Read the model definition and answer for the solid it produces. Units are mm, in the model's axes. Face numbers are marked on the shaded views. Coordinates: 2 decimals unless noted, no trailing zeros. Order: outer loops, then holes, each group sorted by start corner. A loop starts at its lowest first (then second) coordinate and runs counter-clockwise, first axis right, second up. Notation, with made-up numbers: M -6,-27 L 2,-27 A16 ccw 2,-10 Z; hole C 49,79.25 d2. An arc over 180 degrees is marked long. Put each result on its own line as item: value.
Autodesk Inventor part; units mm, degrees
ref_plane "YZ Plane" through (0, 0, 0) normal (1, 0, 0) x (0, 1, 0)
ref_plane "XZ Plane" through (0, 0, 0) normal (0, 1, 0) x (-1, 0, 0)
ref_plane "XY Plane" through (0, 0, 0) normal (0, 0, 1) x (1, 0, 0)
sketch "スケッチ1" plane through (0, 0, 0) normal (0, 1, 0) x (-1, 0, 0)
  circle A0 centre (0, 0) radius 35
  line L0 (0, 0) -> (0, -35)
  line L1 (0, 0) -> (0, 35)
  dimension "d0" = 70
revolve "回転1" add sketch "スケッチ1" angle 180 about axis through (0, 0, 0) along (0, 0, 1) picked at (-2.5961, -23.0408) contours L1 L0 A0
sketch "スケッチ5" plane through (0, 0, 0) normal (0, -1, 0) x (1, 0, 0)
  line L0 (-20, -22) -> (20, -22)
  line L1 (20, -22) -> (20, -13)
  line L2 (20, -13) -> (-20, -13)
  line L3 (-20, -13) -> (-20, -22)
  line L4 (-20, -15) -> (-20, -13)
  line L5 (0, 25) -> (-17, 25)
  line L6 (-17, 25) -> (-17, 23)
  line L7 (-17, 23) -> (0, 23)
  line L8 (0, 23) -> (0, 25)
  line L9 (0, 20) -> (-20, 20)
  line L10 (-20, 20) -> (-20, 19)
  line L11 (-20, 19) -> (0, 19)
  line L12 (0, 19) -> (0, 20)
  line L13 (0, 13) -> (-19, 13)
  line L14 (-19, 13) -> (-19, 11)
  line L15 (-19, 11) -> (0, 11)
  line L16 (0, 11) -> (0, 13)
  line L17 (0, 5) -> (-23, 5)
  line L18 (-23, 5) -> (-23, 3)
  line L19 (-23, 3) -> (0, 3)
  line L20 (0, 3) -> (0, 5)
  circle A0 centre (0, 0) radius 35
  circle A1 centre (0, 0) radius 35
  line L21 (0, 35) -> (0, -35)
  line L22 (35, 0) -> (-35, 0)
  line L23 (-32, 2) -> (-23, 2)
  line L24 (-23, 2) -> (-23, -8)
  line L25 (-23, -8) -> (-32, -8)
  line L26 (-32, -8) -> (-32, 2)
  line L27 (-23, -8.0262) -> (-23, 2)
  line L28 (-27, 22.2711) -> (-27, -22.2711)
  line L29 (-15.5, 25) -> (0, 25)
  line L30 (0, 25) -> (0, 35)
  line L31 (0, 35) -> (-15.5, 35)
  line L32 (-15.5, 35) -> (-15.5, 25)
  line L33 (-15.5, 23) -> (0, 23)
  line L34 (0, 23) -> (0, 20)
  line L35 (0, 20) -> (-15.5, 20)
  line L36 (-15.5, 20) -> (-15.5, 23)
  line L37 (-16, 13) -> (0, 13)
  line L38 (0, 13) -> (0, 19)
  line L39 (0, 19) -> (-16, 19)
  line L40 (-16, 19) -> (-16, 13)
  line L41 (-16, 11) -> (0, 11)
  line L42 (0, 11) -> (0, 5)
  line L43 (0, 5) -> (-16, 5)
  line L44 (-16, 5) -> (-16, 11)
  line L45 (-23, -3) -> (-39.6865, -3)
  line L46 (-23, -3) -> (-7.8337, -3)
  line L47 (-8, 3) -> (-23, 3)
  line L48 (-23, 3) -> (-23, -9)
  line L49 (-23, -9) -> (-8, -9)
  line L50 (-8, -9) -> (-8, 3)
  line L51 (-8, 3) -> (-23, -9) construction
  line L52 (-23, 3) -> (-8, -9) construction
  line L53 (-23, 4) -> (-33, 4)
  line L54 (-33, 4) -> (-33, -10)
  line L55 (-33, -10) -> (-23, -10)
  line L56 (-23, -10) -> (-23, 4)
  line L57 (-23, 4) -> (-33, -10) construction
  line L58 (-33, 4) -> (-23, -10) construction
  line L59 (-8, 3) -> (-1, 3)
  line L60 (-1, 3) -> (-1, -9)
  line L61 (-1, -9) -> (-8, -9)
  line L62 (-8, -9) -> (-8, 3)
  line L63 (-8, 3) -> (-1, -9) construction
  line L64 (-1, 3) -> (-8, -9) construction
  line L65 (-23, 2) -> (-27, 2)
  line L66 (-23, -8) -> (-27, -8)
  line L67 (-23, 4) -> (-27, 4)
  line L68 (-23, -10) -> (-27, -10)
  line L69 (23.4307, -26) -> (-23.4307, -26)
  line L70 (-8, 3) -> (-6.8, 3)
  line L71 (-6.8, 3) -> (-6.8, -9)
  line L72 (-6.8, -9) -> (-8, -9)
  line L73 (-8, -9) -> (-8, 3)
  line L74 (-3, 5) -> (0, 5)
  line L75 (0, 20) -> (-4, 20)
  line L76 (-4, 19) -> (0, 19)
  line L77 (0, 19) -> (0, 20)
  line L78 (-6, 5) -> (-1, 5)
  line L79 (-1, 3) -> (-6, 3)
  point P0 (0, -22)
  point P1 (0, -13)
  point P2 (0, 24)
  point P3 (0, 19.5)
  point P4 (0, 12)
  point P5 (0, 4)
  point P6 (-20, -17.5)
  point P7 (-27, -0.5262)
  point P8 (-27, -8)
  point P9 (-15.5, 21.5)
  point P10 (-15.5, 31.3807)
  point P11 (0, 25)
  point P12 (0, 23)
  point P13 (0, 11)
  point P14 (0, 13)
  point P15 (-27, 0)
  point P16 (-32, 0)
  point P17 (-23, 0)
  point P18 (-15.5, -3)
  point P19 (-28, -3)
  point P20 (-4.5, -3)
  point P21 (-8, -9)
  point P22 (-8, 3)
  point P23 (-27, 0.5)
  point P24 (-28, 0.4738)
  point P25 (-28, -11.5262)
  point P26 (-27, -11.5)
  point P27 (-23, 2)
  point P28 (-23, 2)
  point P29 (-8, 0)
  point P30 (-1, 0)
  point P31 (0, 19)
  point P32 (0, 20)
  point P33 (-27, -10)
  point P34 (-27, 4)
  dimension "d12" = 40
  dimension "d13" = 9
  dimension "d23" = 17
  dimension "d24" = 2
  dimension "d27" = 20
  dimension "d28" = 1
  dimension "d30" = 19
  dimension "d31" = 2
  dimension "d33" = 2
  dimension "d88" = 0
  dimension "d89" = 0
  dimension "d90" = 13
  dimension "d92" = 20
  dimension "d93" = 10
  dimension "d97" = 9
  dimension "d98" = 10
  dimension "d113" = 27
  dimension "d122" = 15.5
  dimension "d123" = 35
  dimension "d124" = 3
  dimension "d125" = 15.5
  dimension "d126" = 6
  dimension "d127" = 6
  dimension "d128" = 16
  dimension "d129" = 16
  dimension "d147" = 12
  dimension "d149" = 8
  dimension "d151" = 15
  dimension "d161" = 14
  dimension "d162" = 10
  dimension "d164" = 12
  dimension "d165" = 7
  dimension "d170" = 26
  dimension "d175" = 1.2
  dimension "d207" = 0
extrude "GNSボード" cut sketch "スケッチ5" against normal blind 16 contours L8 L7 L6 L5
extrude "GNSボード止めるよう" cut sketch "スケッチ5" against normal blind 15 contours L21 L5 L32 A0 | L21 L9 L36 L7
extrude "アルミ板１" cut sketch "スケッチ5" against normal blind 17.5 contours L11 L10 L9 L12
extrude "メイン基板" cut sketch "スケッチ5" against normal blind 17.5 contours L15 L14 L13 L16
extrude "メイン止めるよう" cut sketch "スケッチ5" against normal blind 16.5 contours L17 L44 L15 L21 | L13 L40 L11 L21
extrude "アルミ板２" cut sketch "スケッチ5" against normal blind 19 contours L19 L18 L17 L20
extrude "電池ボックス入れ" cut sketch "スケッチ5" against normal blind 15 contours L3 L2 L21 L0 | L21 L2 L1 L0
extrude "side ut" cut sketch "スケッチ5" against normal blind 100 contours A0 L45 L54 L55 L28 | A0 L22 L54 L45 | L55 L54 L45 L26 L25 L28 | A0 L28 L53 L54 L22 | L54 L22 L26 L45 | L25 L26 L45 L28 | L54 L53 L28 L23 L26 L22 | L26 L22 L28 L45 | L22 L26 L23 L28
extrude "motor case" add sketch "スケッチ5" against normal blind 7 contours L55 L54 L45 L26 L25 L28 | L28 L25 L27 L48 L56 L55 | L50 L46 L24 L22 | L22 L24 L48 L19 L50 | L54 L22 L26 L45 | L28 L45 L24 L25 | L25 L26 L45 L28 | L24 L45 L28 L22 | L22 L28 L23 L24 | L50 L49 L48 L27 L24 L46 | L54 L53 L28 L23 L26 L22 | L26 L22 L28 L45 | L53 L18 L48 L23 L28 | L22 L26 L23 L28
extrude "bottom cut" cut sketch "スケッチ5" against normal blind 90 contours L69 A0 L21 | L21 A0 L69
extrude "motor" cut sketch "スケッチ5" against normal blind 6 contours L60 L61 L71 L22 | L22 L71 L19 L60 | L71 L61 L50 L22 | L22 L50 L19 L71 | L50 L46 L24 L22 | L22 L24 L48 L19 L50 | L28 L45 L24 L25 | L25 L26 L45 L28 | L24 L45 L28 L22 | L22 L28 L23 L24 | L50 L49 L48 L27 L24 L46 | L26 L22 L28 L45 | L22 L26 L23 L28
extrude "motor block" add sketch "スケッチ5" against normal blind 10 contours L71 L61 L50 L22 | L22 L50 L19 L71
sketch "スケッチ27" plane through (-33, 0, -10) normal (-1, 0, 0) x (0, 0, 1)
  line L0 (14, 0) -> (0, 0)
  circle A0 centre (7, 0) radius 3
  point P0 (10, 0)
  dimension "d198" = 6
extrude "押し出し36" cut sketch "スケッチ27" against normal blind 27
mirror "ミラー13" about plane through (0, 0, 0) normal (1, 0, 0) of "メイン止めるよう", "メイン基板", "アルミ板１", "GNSボード止めるよう", "GNSボード", "アルミ板２", "motor", "motor case", "押し出し36", "電池ボックス入れ", "side ut"
ref_plane "作業平面5" through (-17, 17.5, 23) normal (0, -1, 0) x (1, 0, 0)
sketch "スケッチ29" plane through (-17, 17.5, 23) normal (0, -1, 0) x (1, 0, 0)
  line L0 (32.5, 2) -> (1.5, 2)
  line L1 (1.5, 0) -> (32.5, 0)
  line L2 (32.5, -3) -> (1.5, -3)
  line L3 (1, -4) -> (33, -4)
  line L4 (33, -10) -> (1, -10)
  line L5 (33, -10) -> (33, -4)
  line L6 (1, -4) -> (33, -4)
  line L7 (1, -10) -> (1, -4)
  line L8 (1, -12) -> (33, -12)
  line L9 (33, -18) -> (1, -18)
  line L10 (33, -18) -> (33, -12)
  line L11 (1, -12) -> (33, -12)
  line L12 (1, -18) -> (1, -12)
  line L13 (18, -20) -> (40, -20)
  line L14 (-6, -20) -> (17, -20)
  line L15 (17, -18) -> (-6, -18)
  line L16 (-16, -23) -> (-15, -23)
  line L17 (-15, -23) -> (-15, -21)
  line L18 (-15, -21) -> (-6, -21)
  line L19 (-6, -21) -> (-6, -18)
  line L20 (-6, -18) -> (1, -18)
  line L21 (1, -18) -> (1, -12)
  line L22 (1, -12) -> (-2, -12)
  line L23 (-2, -12) -> (-2, -10)
  line L24 (-2, -10) -> (1, -10)
  line L25 (1, -10) -> (1, -4)
  line L26 (1, -4) -> (-3, -4)
  line L27 (-3, -4) -> (-3, -3)
  line L28 (-3, -3) -> (1.5, -3)
  line L29 (1.5, -3) -> (1.5, 0)
  line L30 (1.5, 0) -> (0, 0)
  line L31 (0, 0) -> (0, 2)
  line L32 (0, 2) -> (1.5, 2)
  line L33 (1.5, 2) -> (1.5, 8.3807)
  arc A0 (1.5, 8.3807) -> (-10, -0.7289) centre (17, -23) ccw
  line L34 (-10, -0.7289) -> (-10, -19)
  line L35 (-10, -19) -> (-16, -19)
  line L36 (-16, -19) -> (-16, -23)
  line L37 (49, -23) -> (50, -23)
  line L38 (50, -19) -> (50, -23)
  line L39 (44, -19) -> (50, -19)
  line L40 (44, -19) -> (44, -0.7289)
  arc A1 (44, -0.7289) -> (32.5, 8.3807) centre (17, -23) ccw
  line L41 (32.5, 8.3807) -> (32.5, 2)
  line L42 (32.5, 2) -> (34, 2)
  line L43 (34, 2) -> (34, 0)
  line L44 (34, 0) -> (32.5, 0)
  line L45 (32.5, 0) -> (32.5, -3)
  line L46 (32.5, -3) -> (37, -3)
  line L47 (37, -3) -> (37, -4)
  line L48 (37, -4) -> (33, -4)
  line L49 (33, -4) -> (33, -10)
  line L50 (33, -10) -> (36, -10)
  line L51 (36, -10) -> (36, -12)
  line L52 (36, -12) -> (33, -12)
  line L53 (33, -12) -> (33, -18)
  line L54 (33, -18) -> (40, -18)
  line L55 (40, -18) -> (40, -21)
  line L56 (40, -21) -> (49, -21)
  line L57 (49, -21) -> (49, -23)
  line L58 (40, -18) -> (-6, -18)
  line L59 (-4, -18) -> (38, -18)
  line L60 (38, -18) -> (38, 8.3807)
  line L61 (38, 8.3807) -> (-4, 8.3807)
  line L62 (-4, 8.3807) -> (-4, -18)
  circle A2 centre (17, -23) radius 35
  point P0 (-10, -0.7289)
  point P1 (44, -0.7289)
  point P2 (-4, 5)
  point P3 (38, 5)
  point P4 (37, -3)
  point P5 (38, -18)
  point P6 (32.5, 8.3807)
  point P7 (32.5, 8.3807)
  point P8 (1.5, 8.3807)
  point P9 (1.5, 8.3807)
  dimension "d209" = 2
  dimension "d210" = 2
  dimension "d211" = 26.3807
  dimension "d212" = 70
extrude "押し出し38" cut sketch "スケッチ29" against normal blind 30 contours A1 L40 L39 L38 L37 L57 L56 L55 L54 L60 | L62 L15 L19 L18 L17 L16 L36 L35 L34 A0 | A2 L34 L35 L36 L16 L17 L18 L19 L15 L9 L54 L55 L56 L57 L37 L38 L39 L40
sketch "スケッチ30" plane through (-17, 17.5, 23) normal (0, -1, 0) x (1, 0, 0)
  circle A0 centre (17, -23) radius 50
  line L0 (17, 2) -> (0, 2)
  line L1 (0, 0) -> (17, 0)
  line L2 (-16, -23) -> (-15, -23)
  line L3 (-15, -23) -> (-15, -21)
  line L4 (-15, -21) -> (-6, -21)
  line L5 (-6, -21) -> (-6, -18)
  line L6 (-6, -18) -> (1, -18)
  line L7 (1, -18) -> (1, -12)
  line L8 (1, -12) -> (-2, -12)
  line L9 (-2, -12) -> (-2, -10)
  line L10 (-2, -10) -> (1, -10)
  line L11 (1, -10) -> (1, -4)
  line L12 (1, -4) -> (-3, -4)
  line L13 (-3, -4) -> (-3, -3)
  line L14 (-3, -3) -> (1.5, -3)
  line L15 (1.5, -3) -> (1.5, 0)
  line L16 (1.5, 0) -> (0, 0)
  line L17 (0, 0) -> (0, 2)
  line L18 (0, 2) -> (1.5, 2)
  line L19 (1.5, 2) -> (1.5, 8.3807)
  arc A1 (1.5, 8.3807) -> (-10, -0.7289) centre (17, -23) ccw
  line L20 (-10, -0.7289) -> (-10, -19)
  line L21 (-10, -19) -> (-16, -19)
  line L22 (-16, -19) -> (-16, -23)
  line L23 (-4, -18) -> (-4, -1.1425)
  dimension "d215" = 100
  dimension "d218" = 5
extrude "押し出し39" cut sketch "スケッチ30" along normal blind 100 contours A0 | L0 L17 L1 L15 L14 L13 L12 L11 L10 L9 L8 L7 L6 L5 L4 L3 L2 L22 L21 L20 A1 L19
sketch "スケッチ31" plane through (0, 17.5, 0) normal (0, -1, 0) x (1, 0, 0)
  line L0 (-16, 5) -> (-16, 11)
  line L1 (-19, 11) -> (0, 11)
  line L2 (-19, 13) -> (-19, 11)
  line L3 (0, 13) -> (-19, 13)
  line L4 (-16, 19) -> (-16, 13)
  line L5 (-20, 19) -> (0, 19)
  line L6 (0, 20) -> (-20, 20)
  line L7 (-16, 11) -> (-21, 5)
  line L8 (-21, 5) -> (-16, 5)
  line L9 (21, 5) -> (-21, 5)
  line L10 (-21, 5) -> (-21, 21.8575)
  line L11 (-21, 11) -> (-16, 5)
  line L12 (-16, 11) -> (-21, 11)
  circle A0 centre (-18.5, 8) radius 1.5
  point P0 (0, 0)
  dimension "d219" = 3
extrude "押し出し40" cut sketch "スケッチ31" against normal blind 100 contours A0 L7 L11 | L11 L7 A0 | L7 L11 A0 | A0 L11 L7
properties part number "body back for main 2" material "ABS プラスチック"
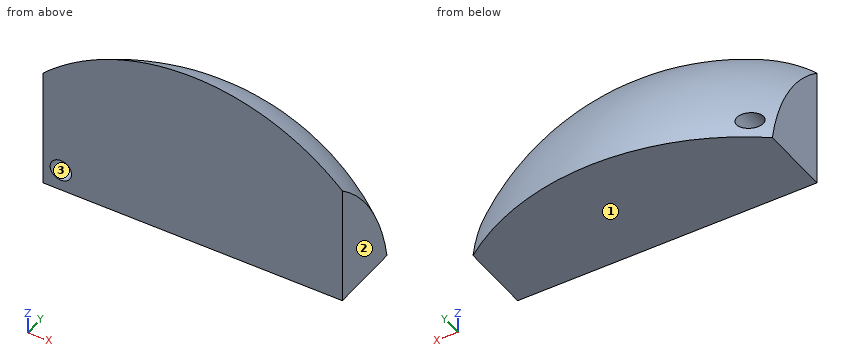
Q1. Find section A-A on x = -18.5. Write down the section's boundary in (y, z), plus the area to 3 significant figures.
Answers below:
outline: M 17.5,5 L 29.29,5 A29.71 ccw 28.99,6.5 L 17.5,6.5 Z; M 17.5,9.5 L 28.15,9.5 A29.71 ccw 17.5,24.01 Z
area: 112 mm^2
Q2. Consider line 1 along X through (y, z) = (21.25, 8); line 2 along Z through (x, y) = (-18.5, 24); line 3 along Z through (x, y) = (-18.5, 21.75). Determine where each line is inside the solid, lowest interval first.
Answers below:
line 1: x = -21 to -20, -17 to 21
line 2: z = 5 to 6.5, 9.5 to 17.51
line 3: z = 5 to 6.5, 9.5 to 20.24
Q3. Given pin 1 (4 mm diameter, centred on x = -18.5, z = 8, fed in from +Y); pin 2 (4 mm diameter, centred on x = 4, z = 19.5, fed in from +Y); pin 3 (5 mm diameter, centred on y = 26, z = 16, fed in from +X), each flat-ended and moving along its own axis, determine where each tip first touches the part or whether it passes through.
Answers below:
pin 1: stops at y = 29.92
pin 2: stops at y = 30.07
pin 3: stops at x = 20.96
Q4. For a pull along Z with two mould halves and no side action, classify the marked faces 1, 2 and 3 as +Z half, -Z half, draft (parallel to the pull), parting line (faces both ways), or undercut.
Answers below:
face 1: -Z half
face 2: draft
face 3: undercut
Q5. Find section D-D on y = 28.25. Write down the section's boundary in (x, z), plus the area to 3 significant figures.
Answers below:
outline: M -20.05,5 L 20.05,5 A20.66 ccw -18.35,9.49 A1.5 cw long -19.49,6.87 A20.66 ccw Z
area: 461 mm^2
Q6. Find section B-B on y = 24. Write down the section's boundary in (x, z), plus the area to 3 significant figures.
Answers below:
outline: M -21,5 L 21,5 L 21,14.42 A25.48 ccw -21,14.42 Z; hole C -18.5,8 d3
area: 715 mm^2
Q7. Find section C-C on z = 23.25. Write down the section's boundary in (x, y).
Answers below:
outline: M -19.45,17.5 L 19.45,17.5 A26.16 ccw Z
